```python
from build123d import *
from OCP.BRepFilletAPI import BRepFilletAPI_MakeChamfer
from build123d.topology import SkipClean

# Parameters (mm, degrees)
SKETCH1_R           = 40
SKETCH1_R_2         = 20
BOSS_EXTRUDE1_DEPTH = 8
BOSS_EXTRUDE2_START = 12
SKETCH3_R           = 20
BOSS_EXTRUDE2_DEPTH = 12
SKETCH5_R           = 7.5
CUT_EXTRUDE3_DEPTH  = 10
SKETCH2_R           = 4
CUT_EXTRUDE1_DEPTH  = 20
BOSS_EXTRUDE3_DEPTH = 8
CHAMFER1_SIZE       = 19.800694827
CHAMFER1_SIZE_2     = 8
BOSS_EXTRUDE4_DEPTH = 12
FILLET1_R           = 6
CUT_EXTRUDE4_DEPTH  = 6
SKETCH9_R           = 4.2
CUT_EXTRUDE5_DEPTH  = 6
CUT_EXTRUDE7_START  = -12
CUT_EXTRUDE7_DEPTH  = 12


with BuildPart() as part:
    # Sketch1 → Boss-Extrude1 (new body)
    with BuildSketch(Plane(origin=(0, 0, 0), x_dir=(1, 0, 0), z_dir=(0, 1, 0))):
        with Locations(Location((0, 0, 0), (0, 0, 270))):
            Circle(SKETCH1_R)
        with Locations(Location((0, 0, 0), (0, 0, 270))):
            Circle(SKETCH1_R_2, mode=Mode.SUBTRACT)
    extrude(amount=BOSS_EXTRUDE1_DEPTH)

    # Sketch3 → Boss-Extrude2 (add)
    with SkipClean():  # the faces are left unmerged after this step: merging them gives an invalid solid
        with BuildSketch(Plane.XZ.offset(BOSS_EXTRUDE2_START)):
            with BuildLine():
                Line((20.894189842, 56.244402662), (105, 25))
                Line((105, 25), (105, -25))
                Line((105, -25), (20.894189842, -56.244402662))
                ThreePointArc((20.894189842, -56.244402662), (-60, 0), (20.894189842, 56.244402662))
            make_face()
            with Locations(Location((0, 0, 0), (0, 0, 270))):
                Circle(SKETCH3_R, mode=Mode.SUBTRACT)
        extrude(amount=-BOSS_EXTRUDE2_DEPTH)

    # Sketch5 → Cut-Extrude3 (cut)
    with SkipClean():  # the faces are left unmerged after this step: merging them gives an invalid solid
        with BuildSketch(Plane.XZ.offset(12)):
            with Locations(Location((0, 30, 0), (0, 0, 270))):
                Circle(SKETCH5_R)
            with Locations(Location((30, 0, 0), (0, 0, 270))):
                Circle(SKETCH5_R)
            with Locations(Location((0, -30, 0), (0, 0, 270))):
                Circle(SKETCH5_R)
            with Locations(Location((-30, 0, 0), (0, 0, 270))):
                Circle(SKETCH5_R)
        extrude(amount=-CUT_EXTRUDE3_DEPTH, mode=Mode.SUBTRACT)

    # Sketch2 → Cut-Extrude1 (cut)
    with SkipClean():  # the faces are left unmerged after this step: merging them gives an invalid solid
        with BuildSketch(Plane(origin=(0, 8, 0), x_dir=(1, 0, 0), z_dir=(0, 1, 0))):
            with Locations(Location((30, 0, 0), (0, 0, 270))):
                Circle(SKETCH2_R)
            with Locations(Location((0, -30, 0), (0, 0, 270))):
                Circle(SKETCH2_R)
            with Locations(Location((-30, 0, 0), (0, 0, 270))):
                Circle(SKETCH2_R)
            with Locations(Location((0, 30, 0), (0, 0, 270))):
                Circle(SKETCH2_R)
        extrude(amount=-CUT_EXTRUDE1_DEPTH, mode=Mode.SUBTRACT)

    # Sketch6 → Boss-Extrude3 (add)
    with SkipClean():  # the faces are left unmerged after this step: merging them gives an invalid solid
        with BuildSketch(Plane(origin=(0, 0, 0), x_dir=(1, 0, 0), z_dir=(0, 1, 0))):
            with BuildLine():
                Line((-7.5, -39.290584114), (-7.5, -59.529404499))
                ThreePointArc((-7.5, -59.529404499), (0, -60), (7.5, -59.529404499))
                Line((7.5, -59.529404499), (7.5, -39.290584114))
                ThreePointArc((7.5, -39.290584114), (0, -40), (-7.5, -39.290584114))
            make_face()
            with BuildLine():
                Line((-39.290584114, -7.5), (-59.529404499, -7.5))
                ThreePointArc((-59.529404499, -7.5), (-60, 0), (-59.529404499, 7.5))
                Line((-59.529404499, 7.5), (-39.290584114, 7.5))
                ThreePointArc((-39.290584114, 7.5), (-40, 0), (-39.290584114, -7.5))
            make_face()
            with BuildLine():
                Line((-7.5, 39.290584114), (-7.5, 59.529404499))
                ThreePointArc((-7.5, 59.529404499), (0, 60), (7.5, 59.529404499))
                Line((7.5, 59.529404499), (7.5, 39.290584114))
                ThreePointArc((7.5, 39.290584114), (0, 40), (-7.5, 39.290584114))
            make_face()
            with BuildLine():
                Line((39.290584114, 7.5), (59.529404499, 7.5))
                ThreePointArc((59.529404499, 7.5), (60, 0), (59.529404499, -7.5))
                Line((59.529404499, -7.5), (39.290584114, -7.5))
                ThreePointArc((39.290584114, -7.5), (40, 0), (39.290584114, 7.5))
            make_face()
        extrude(amount=BOSS_EXTRUDE3_DEPTH)

    # Chamfer1
    chamfer1_edges_1 = [part.edges().sort_by_distance(p)[0] for p in [
        (0, 8, -60),
    ]]
    chamfer1_side_1 = [part.faces().sort_by_distance(p)[0] for p in [
        (0, 8, -59.84),
    ]]
    chamfer1_edges_2 = [part.edges().sort_by_distance(p)[0] for p in [
        (60, 8, 0),
    ]]
    chamfer1_side_2 = [part.faces().sort_by_distance(p)[0] for p in [
        (60, 7.84, 0),
    ]]
    chamfer1_edges_3 = [part.edges().sort_by_distance(p)[0] for p in [
        (0, 8, 60),
    ]]
    chamfer1_side_3 = [part.faces().sort_by_distance(p)[0] for p in [
        (0, 8, 59.84),
    ]]
    chamfer1_edges_4 = [part.edges().sort_by_distance(p)[0] for p in [
        (-60, 8, 0),
    ]]
    chamfer1_side_4 = [part.faces().sort_by_distance(p)[0] for p in [
        (-59.84, 8, 0),
    ]]
    chamfer1 = BRepFilletAPI_MakeChamfer(part.part.solid().wrapped)
    for e in chamfer1_edges_1:
        chamfer1.Add(CHAMFER1_SIZE - 0.0001, CHAMFER1_SIZE_2 - 0.0001, e.wrapped, chamfer1_side_1[0].wrapped)
    for e in chamfer1_edges_2:
        chamfer1.Add(CHAMFER1_SIZE_2 - 0.0001, CHAMFER1_SIZE - 0.0001, e.wrapped, chamfer1_side_2[0].wrapped)
    for e in chamfer1_edges_3:
        chamfer1.Add(CHAMFER1_SIZE - 0.0001, CHAMFER1_SIZE_2 - 0.0001, e.wrapped, chamfer1_side_3[0].wrapped)
    for e in chamfer1_edges_4:
        chamfer1.Add(CHAMFER1_SIZE - 0.0001, CHAMFER1_SIZE_2 - 0.0001, e.wrapped, chamfer1_side_4[0].wrapped)
    add(Compound.cast(chamfer1.Shape()), mode=Mode.REPLACE)  # a hair under: the kernel refuses the full size

    # Sketch7 → Boss-Extrude4 (add)
    with BuildSketch(Plane.XZ.offset(12)):
        with BuildLine():
            Line((115, 12.5), (105, 12.5))
            Line((105, 12.5), (105, -12.5))
            Line((105, -12.5), (115, -12.5))
            ThreePointArc((115, -12.5), (127.5, 0), (115, 12.5))
        make_face()
    extrude(amount=-BOSS_EXTRUDE4_DEPTH)

    # Fillet1
    fillet1_edges = [part.edges().sort_by_distance(p)[0] for p in [
        (105, -6, -25),
        (105, -6, 25),
        (105, -6, -12.5),
        (105, -6, 12.5),
    ]]
    fillet(fillet1_edges, radius=FILLET1_R)

    # Sketch8 → Cut-Extrude4 (cut)
    with BuildSketch(Plane.XZ.offset(12)):
        Polygon((111.24722325, -6.5), (118.75277675, -6.5), (122.505553499, 0), (118.75277675, 6.5), (111.24722325, 6.5), (107.494446501, 0), align=None)
    extrude(amount=-CUT_EXTRUDE4_DEPTH, mode=Mode.SUBTRACT)

    # Sketch9 → Cut-Extrude5 (cut)
    with BuildSketch(Plane.XZ.offset(6)):
        with Locations(Location((115, 0, 0), (0, 0, 270))):
            Circle(SKETCH9_R)
    extrude(amount=-CUT_EXTRUDE5_DEPTH, mode=Mode.SUBTRACT)

    # Sketch11 → Cut-Extrude7 (cut)
    with BuildSketch(Plane(origin=(0, 0, 0), x_dir=(1, 0, 0), z_dir=(0, 1, 0)).offset(CUT_EXTRUDE7_START)):
        with BuildLine():
            Line((93, 20.923688206), (93, 13.5))
            Line((93, 13.5), (58.46152581, 13.5))
            ThreePointArc((58.46152581, 13.5), (53.766674065, 26.62977206), (46.167935821, 38.321295672))
            Line((46.167935821, 38.321295672), (93, 20.923688206))
        make_face()
    cut_extrude7 = extrude(amount=CUT_EXTRUDE7_DEPTH, mode=Mode.SUBTRACT)

    # Mirror1: Cut-Extrude7 across plane
    add(cut_extrude7.mirror(Plane.XY), mode=Mode.SUBTRACT)


solid = part.part
```
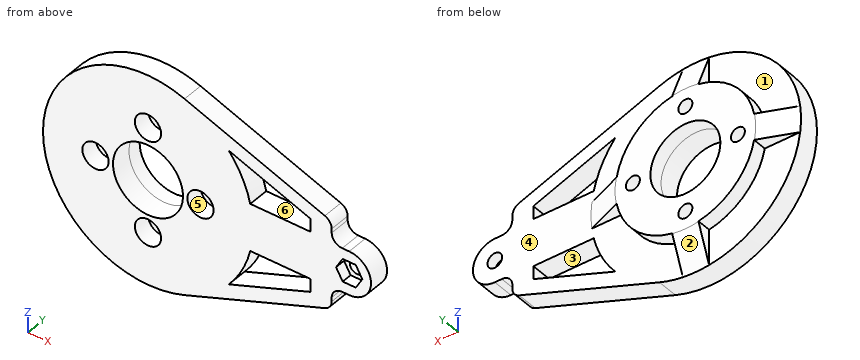
Source: CAD feature listing. Evaluate the final solid. Frame: model axes, mm. Face numbers are marked on the shaded views. A direction names the side the tool comes from. Give positions to 0.01 mm unless a question says otherwise; leave off trailing zeros. Loops run counter-clockwise (first coordinate to the right, second up) from the corner with the lowest first, then second, coordinate; pieces in that order, holes last. Notation, with made-up numbers: M -18,33 L 13,33 A14 ccw 13,46 Z; hole C -30.75,9 d5. An arc over 180 degrees is marked long. Put each result on its own line as item: value.
Q1. Pin query (flat end, axial travel): P1, Ø8, axis at x = 71.5, z = 16.5, coming from the +Y side; P2, Ø4, axis at y = 4.5, z = -47.5, coming from the +X side; P3, Ø4.5, axis at x = -1.5, z = -27, coming from the -Y side; P4, Ø7, axis at x = 0, z = -30, coming from the +Y side. Return the tip coordinate at first contact, or that it passes through.
Response values:
P1: stops at y = 0
P2: stops at x = 7.5
P3: stops at y = -2
P4: passes through
Q2. Section C-C (y = 3.5). Return the cut outline in (x, z).
Response values:
outline: M -50.79,-7.5 L -39.29,-7.5 A40 ccw -7.5,-39.29 L -7.5,-50.79 A51.34 ccw 7.5,-50.79 L 7.5,-39.29 A40 ccw 39.29,-7.5 L 50.79,-7.5 A51.34 ccw 50.79,7.5 L 39.29,7.5 A40 ccw 7.5,39.29 L 7.5,50.79 A51.34 ccw -7.5,50.79 L -7.5,39.29 A40 ccw -39.29,7.5 L -50.79,7.5 A51.34 ccw Z; hole C -30,0 d8; hole C 0,0 d40; hole C 0,-30 d8; hole C 0,30 d8; hole C 30,0 d8
Q3. Section A-A (x = 0). Return the cut outline in (y, z), and give its area (3 significant figures).
Response values:
outline: M -12,-60 L 0,-60 L 8,-40.2 L 8,-34 L -2,-34 L -2,-37.5 L -12,-37.5 Z; M -12,-22.5 L -2,-22.5 L -2,-26 L 8,-26 L 8,-20 L -12,-20 Z; M -12,20 L 8,20 L 8,26 L -2,26 L -2,22.5 L -12,22.5 Z; M -12,37.5 L -2,37.5 L -2,34 L 8,34 L 8,40.2 L 0,60 L -12,60 Z
area: 982 mm²
Q4. Reachability of the marked faces 4, 5 and 6 from +Z, -Z, +X, -X, +Y, -Y: full face, straight path, thin tool, end or side. Return the list, or none.
Response values:
face 4: +X, +Y
face 5: -Y
face 6: +Y, -Y
Q5. Mould query, pull axis Z, two halves, no side actions, for the marked faces 1, 2 and 3. Classes: released by +Z, released by -Z, zero draft, split by the parting line, or undercut.
Response values:
face 1: zero draft
face 2: released by -Z
face 3: undercut
Q6. Section B-B (z = -30). Return the cut outline in (x, y).
Response values:
outline: M -51.96,-12 L -7.5,-12 L -7.5,-2 L -4,-2 L -4,8 L -26.46,8 L -26.46,0 L -51.96,0 Z; M 4,-2 L 7.5,-2 L 7.5,-12 L 51.96,-12 L 51.96,0 L 26.46,0 L 26.46,8 L 4,8 Z; M 68.57,-12 L 91.54,-12 L 91.54,0 L 68.57,0 Z
Q7. Line query: probe 1 along X at (y, z) = (5.5, 0); probe 2 along Y at (x, z) = (34, -26); probe 3 along Y at (x, z) = (27, -4). Output: solid intervals per line, ascending. Write a range as [from, to].
Response values:
probe 1: x = [-46.39, -34], [-26, -20], [20, 26], [34, 46.39]
probe 2: y = [-12, 0]
probe 3: y = [-2, 8]
Q8. Section D-D (x = 66.5). Return the cut outline in (y, z), and give its area (3 significant figures).
Response values:
outline: M -12,-39.3 L 0,-39.3 L 0,-30.77 L -12,-30.77 Z; M -12,-13.5 L 0,-13.5 L 0,13.5 L -12,13.5 Z; M -12,30.77 L 0,30.77 L 0,39.3 L -12,39.3 Z
area: 529 mm²
